Input: part model. Units: mm. Frame: model coordinates. Face numbers are marked on the shaded views. A direction names the side the tool comes from. Coordinates: 2 decimals unless noted, no trailing zeros. Loops run counter-clockwise (first coordinate to the right, second up) from the corner with the lowest first, then second, coordinate; pieces in that order, holes last. Notation, with made-up numbers: (21.5, -21.5) - (34.5, -21.5) arc R13 cw to (34.5, -10.5) - close; hole circle Ø7 at (86.5, 16). An arc over 180 degrees is marked (long way). Use one line per item in the form item = value.
Autodesk Inventor part; units mm, degrees
ref_plane "YZ Plane" through (0, 0, 0) normal (1, 0, 0) x (0, 1, 0)
ref_plane "XZ Plane" through (0, 0, 0) normal (0, 1, 0) x (-1, 0, 0)
ref_plane "XY Plane" through (0, 0, 0) normal (0, 0, 1) x (1, 0, 0)
sketch "草图1" plane through (0, 0, 0) normal (0, 1, 0) x (-1, 0, 0)
  circle A0 centre (0, 0) radius 10
  dimension "d0" = 20
extrude "拉伸1" add sketch "草图1" against normal blind 5
fillet "圆角1" radius 2 1 edges at (10, 0, 0)
shell "抽壳1" thickness 1.5 removed faces 1 at (1.182, -5, 3.1167)
move or copy body "旋转1" bodies to move or copy 1 copy no rotation origin (0, 0, 0) rotation axis (1, 0, 0) rotation angle 90 translate (0, -1.5, 1.5)
properties part number "Buttonx20" material "玻璃"
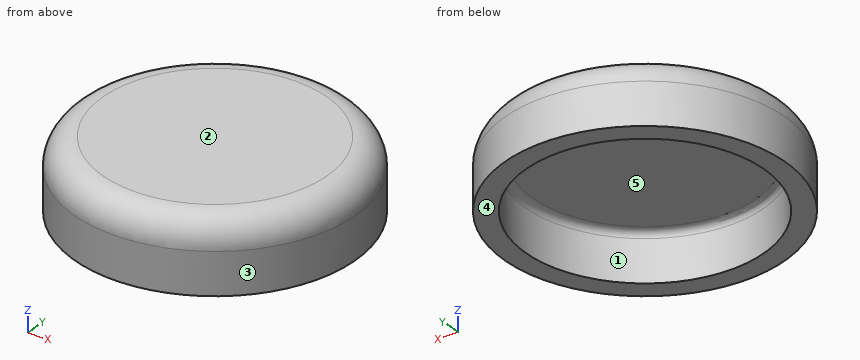
Q1. Set-up query: the marked faces 4 and 5. Return all of +Z, -Z, +X, -X, +Y, -Y with unobstructed straight access to the full face (end or side cutting, diameter ignored); none if empty.
Check values:
face_4 = -Z, +X, -X, +Y, -Y
face_5 = -Z
Q2. First-contact query: P1, Ø1.5, axis at x = -4, z = 0.5, coming from the +Y side; P2, Ø2, axis at x = 0, y = 3.5, coming from the -Z side; P3, Ø1.5, axis at x = 0.5, z = -2.5, coming from the -Y side. Flat tips, straight axial feed; report the tip coordinate or a pass-through.
Check values:
P1 = 7.82
P2 = 0
P3 = -11.5
Q3. Cut plane A-A, the plane y = -1.5. Return loops of the section in (x, z), then the cut area to 3 significant figures.
Check values:
outline = (-10, -3.5) - (-8.5, -3.5) - (-8.5, -0.5) arc R0.5 cw to (-8, 0) - (8, 0) arc R0.5 cw to (8.5, -0.5) - (8.5, -3.5) - (10, -3.5) - (10, -0.5) arc R2 ccw to (8, 1.5) - (-8, 1.5) arc R2 ccw to (-10, -0.5) - close
area = 38.9 mm²
Q4. Cut plane B-B, the plane z = -2.9. Return loops of the section in (x, y).
Check values:
outline = circle Ø20 at (0, -1.5); hole circle Ø17 at (0, -1.5)
Q5. Pull-direction query (Y, two-part tool) for the marked faces 1, 2 and 3; classes: pulls with the +Y half, pulls with the -Y half, needs draft (parallel to the pull), parting line crosses it, or undercut.
Check values:
face_1 = undercut
face_2 = needs draft
face_3 = parting line crosses it
Q6. Cut plane C-C, the plane x = 0. Return loops of the section in (y, z).
Check values:
outline = (-11.5, -3.5) - (-10, -3.5) - (-10, -0.5) arc R0.5 cw to (-9.5, 0) - (6.5, 0) arc R0.5 cw to (7, -0.5) - (7, -3.5) - (8.5, -3.5) - (8.5, -0.5) arc R2 ccw to (6.5, 1.5) - (-9.5, 1.5) arc R2 ccw to (-11.5, -0.5) - close
Q7. Ray query, line 1 along Y through (x, z) = (0, -2.4); line 2 along X through (y, z) = (-1.5, -2.9); line 3 along Z through (x, y) = (3, -0.5). Return the intervals inside material, ascending. Write a range as [from, to].
Check values:
line_1 = [-11.5, -10], [7, 8.5]
line_2 = [-10, -8.5], [8.5, 10]
line_3 = [0, 1.5]
